```python
from build123d import *

# Parameters (mm, degrees)
BOSS_EXTRUDE1_DEPTH     = 17
CUT_EXTRUDE1_DEPTH      = 34.119329703
CUT_EXTRUDE1_DEPTH_BACK = 34.119329703
SKETCH2_R               = 12.8
SKETCH3_R               = 2
CUT_EXTRUDE2_DEPTH      = 7.5


with BuildPart() as part:
    # Sketch1 → Boss-Extrude1 (new, symmetric)
    with BuildSketch(Plane(origin=(0, 0, 0), x_dir=(0, 0, -1), z_dir=(1, 0, 0))):
        with BuildLine():
            Line((-19, 0.6), (19, 0.6))
            ThreePointArc((19, 0.6), (21.828427125, 1.771572875), (23, 4.6))
            Line((23, 4.6), (23, 12.7))
            ThreePointArc((23, 12.7), (21.828427125, 15.528427125), (19, 16.7))
            Line((19, 16.7), (-19, 16.7))
            ThreePointArc((-19, 16.7), (-21.828427125, 15.528427125), (-23, 12.7))
            Line((-23, 12.7), (-23, 4.6))
            ThreePointArc((-23, 4.6), (-21.828427125, 1.771572875), (-19, 0.6))
        make_face()
    extrude(amount=BOSS_EXTRUDE1_DEPTH, both=True)

    # Sketch2 → Cut-Extrude1 (cut, two sides: drawn at the far end of the back side and taken through both)
    with BuildSketch(Plane(origin=(0, 0, 0), x_dir=(0, 0, -1), z_dir=(1, 0, 0)).offset(-CUT_EXTRUDE1_DEPTH_BACK)):
        Circle(SKETCH2_R)
    extrude(amount=CUT_EXTRUDE1_DEPTH + CUT_EXTRUDE1_DEPTH_BACK, mode=Mode.SUBTRACT)

    # Sketch3 → Cut-Extrude2 (cut)
    with BuildSketch(Plane(origin=(0, 0.6, 0), x_dir=(1, 0, 0), z_dir=(0, 1, 0))):
        with Locations(Location((12, -17.5, 0), (0, 0, 228.590377891))):
            Circle(SKETCH3_R)
        with Locations(Location((12, 17.5, 0), (0, 0, 48.590377891))):
            Circle(SKETCH3_R)
        with Locations(Location((-12, -17.5, 0), (0, 0, 228.590377891))):
            Circle(SKETCH3_R)
        with Locations(Location((-12, 17.5, 0), (0, 0, 48.590377891))):
            Circle(SKETCH3_R)
    extrude(amount=CUT_EXTRUDE2_DEPTH, mode=Mode.SUBTRACT)


solid = part.part
```
Work out the finished part from the listing and answer in its coordinate system (mm). A direction names the side the tool comes from. Give positions to 0.01 mm unless a question says otherwise; leave off trailing zeros. Loops run counter-clockwise (first coordinate to the right, second up) from the corner with the lowest first, then second, coordinate; pieces in that order, holes last. Notation, with made-up numbers: (56, -7.75) - (101, -7.75) arc R6 cw to (101, -1.75) - close; hole circle Ø6 at (6, -12). An arc over 180 degrees is marked (long way). One line per question, with ' | ' between items.
(1) Straight lines are drawn through the part: probe 1 along X at (y, z) = (3.5, -17.5); probe 2 along Z at (x, y) = (-12, 5.25); probe 3 along X at (y, z) = (1.75, 17). For each, find the intervals that lie inside material, in ascending order.
Recorded:
probe 1: x = -17 to -14, -10 to 10, 14 to 17 | probe 2: z = -23 to -19.5, -15.5 to -11.67, 11.67 to 15.5, 19.5 to 23 | probe 3: x = -17 to -13.94, -10.06 to 10.06, 13.94 to 17
(2) The part is cut by section C-C (z = 17.5). Write down the section's boundary in (x, y).
Recorded:
outline: (-17, 0.6) - (-14, 0.6) - (-14, 8.1) - (-10, 8.1) - (-10, 0.6) - (10, 0.6) - (10, 8.1) - (14, 8.1) - (14, 0.6) - (17, 0.6) - (17, 16.7) - (-17, 16.7) - close
(3) The mould has two halves that part along X. Classify faces 1 (the face through (10.203, 4.297, 18.379)), 2 (the face through (-0.238, 12.797, -0.273)), 3 (the face through (17, 14, 0)): +X half, -X half, draft (parallel to the pull), parting line (faces both ways), or undercut.
Recorded:
face 1: undercut | face 2: draft | face 3: +X half
(4) The part is cut by section A-A (y = 9.75). Write down the section's boundary in (x, z), then the cut area to 3 significant figures.
Recorded:
outline: (-17, -23) - (17, -23) - (17, -8.29) - (-17, -8.29) - close; (-17, 8.29) - (17, 8.29) - (17, 23) - (-17, 23) - close | area: 1,000 mm²
(5) The part is cut by section B-B (x = -7). Write down the section's boundary in (y, z).
Recorded:
outline: (0.6, -19) arc R4 ccw to (4.6, -23) - (12.7, -23) arc R4 ccw to (16.7, -19) - (16.7, 19) arc R4 ccw to (12.7, 23) - (4.6, 23) arc R4 ccw to (0.6, 19) - (0.6, 12.79) arc R12.8 cw to (0.6, -12.79) - close
(6) Each of these flat-tipped pins is pushed along its axis until it touches: pin 1 Ø4.5 at (x, z) = (13, 17.5) entering from -Y; pin 2 Ø3 at (x, z) = (12, -17.5) entering from -Y; pin 3 Ø1 at (x, z) = (-6, 0.5) entering from -Y; pin 4 Ø2 at (x, y) = (13.5, 14.5) entering from -Z. Where does it stop, or does it pass through?
Recorded:
pin 1: stops at y = 0.6 | pin 2: stops at y = 8.1 | pin 3: stops at y = 12.76 | pin 4: stops at z = -22.92
(7) A tool of negligible diameter and unlimited length cuts with its end or side. For faces 4 (the face through (0, 9, -23)), 5 (the face through (-13.797, 4.297, 18.379)), from which of +Z, -Z, +X, -X, +Y, -Y can it reach the whole face along a straight path? Write none if from no direction.
Recorded:
face 4: -Z, +X, -X, +Y, -Y | face 5: -Y
(8) The part is cut by section D-D (x = -12). Write down the section's boundary in (y, z).
Recorded:
outline: (0.6, -15.5) - (8.1, -15.5) - (8.1, -19.5) - (0.63, -19.5) arc R4 ccw to (4.6, -23) - (12.7, -23) arc R4 ccw to (16.7, -19) - (16.7, 19) arc R4 ccw to (12.7, 23) - (4.6, 23) arc R4 ccw to (0.63, 19.5) - (8.1, 19.5) - (8.1, 15.5) - (0.6, 15.5) - (0.6, 12.79) arc R12.8 cw to (0.6, -12.79) - close
